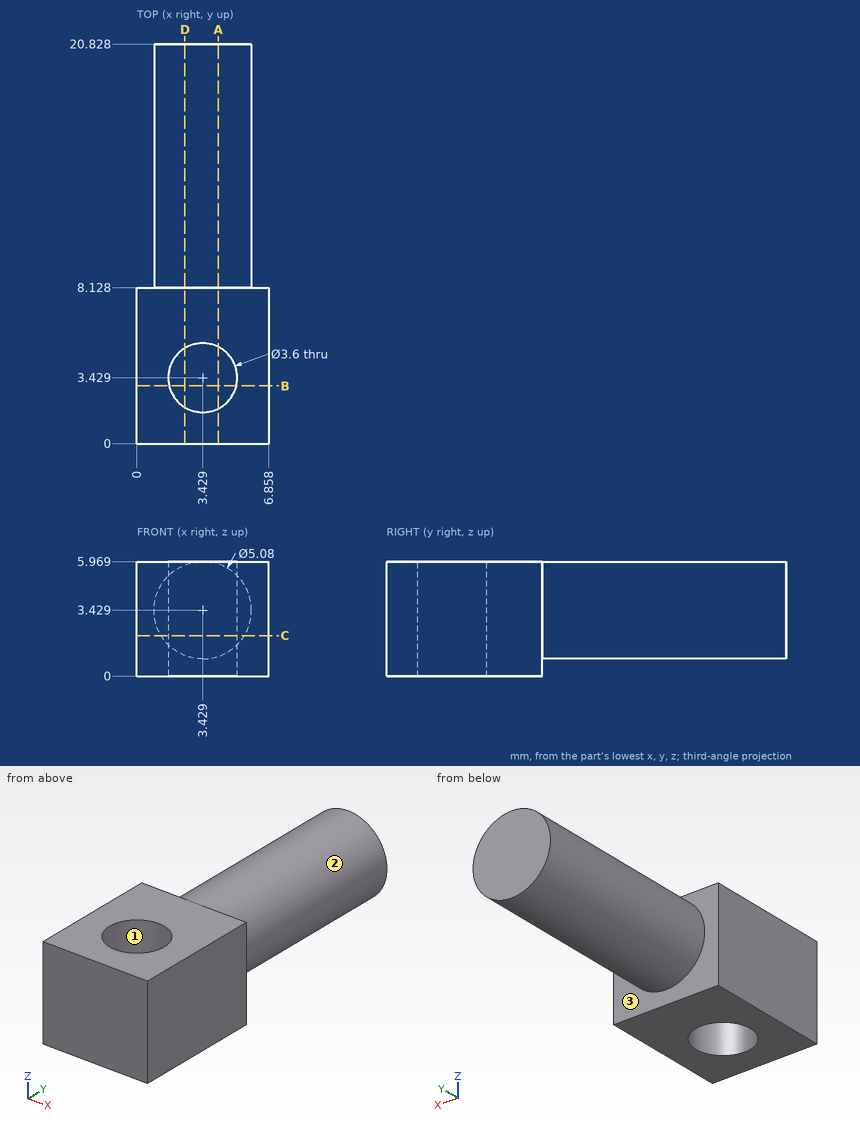
For this review, use the dimensioned drawing (mm, ordinates from the lowest corner) and the shaded views. Round coordinates to 2 decimals unless told otherwise and drop trailing zeros. Order: outer loops, then holes, each group sorted by start corner. A loop starts at its lowest first (then second) coordinate and runs counter-clockwise, first axis right, second up. Notation, with made-up numbers: (-10, 33.25) -> (38, 33.25) arc R22 ccw to (38, 70.25) -> close; hole circle Ø6 at (74.5, 53.5). An arc over 180 degrees is marked (long way). One line per item, written item: value. Start each with the question number.
Q1. Take a section at B-B (y = 3). Write out the cut boundary in (x, z).
Q2. Clearance check with flat-ended pins moving along their axes: pin 1 Ø4 at (x, y) = (4.5, 10) entering from +Z; pin 2 Ø2 at (x, y) = (5, 16.5) entering from -Z; pin 3 Ø1.5 at (y, z) = (17.5, 4.5) entering from +X; pin 4 Ø2 at (x, y) = (1.5, 10) entering from -Z (3 decimals). State where each tip first meets the part, or that it passes through.
Q3. Take a section at D-D (x = 2.5). Write out the cut boundary in (y, z).
Q4. Mouldability with a two-part tool opening along X and no side actions: class the marked faces 1, 2 and 3 as released by +X, released by -X, zero draft, split by the parting line, or undercut.
Q5. Take a section at A-A (x = 4.25). Write out the cut boundary in (y, z), and give its area (3 significant figures).
Q6. Take a section at C-C (z = 2.1). Write out the cut boundary in (x, y), and give its area (3 significant figures).
Q7. Wall thickness on line 1 (X direction, y = 3.5, z = 5.65); line 2 (Y direction, x = 0.5, z = 1.55); line 3 (Y direction, x = 4, z = 3.05): over which ranges is each line inside the solid? List them lowest first.
Reported:
1. outline: (0, 0) -> (1.68, 0) -> (1.68, 5.97) -> (0, 5.97) -> close; (5.18, 0) -> (6.86, 0) -> (6.86, 5.97) -> (5.18, 5.97) -> close
2. pin 1: stops at z = 5.97
2. pin 2: stops at z = 0.95
2. pin 3: stops at x = 5.95
2. pin 4: stops at z = 1.065
3. outline: (0, 0) -> (1.89, 0) -> (1.89, 5.97) -> (0, 5.97) -> close; (4.97, 0) -> (8.13, 0) -> (8.13, 1.06) -> (20.83, 1.06) -> (20.83, 5.79) -> (8.13, 5.79) -> (8.13, 5.97) -> (4.97, 5.97) -> close
4. face 1: undercut
4. face 2: split by the parting line
4. face 3: zero draft
5. outline: (0, 0) -> (1.83, 0) -> (1.83, 5.97) -> (0, 5.97) -> close; (5.03, 0) -> (8.13, 0) -> (8.13, 1.03) -> (20.83, 1.03) -> (20.83, 5.83) -> (8.13, 5.83) -> (8.13, 5.97) -> (5.03, 5.97) -> close
5. area: 90.4 mm2
6. outline: (0, 0) -> (6.86, 0) -> (6.86, 8.13) -> (5.59, 8.13) -> (5.59, 20.83) -> (1.26, 20.83) -> (1.26, 8.13) -> (0, 8.13) -> close; hole circle Ø3.6 at (3.43, 3.43)
6. area: 101 mm2
7. line 1: x = 0 to 1.63, 5.23 to 6.86
7. line 2: y = 0 to 8.13
7. line 3: y = 0 to 1.72, 5.14 to 20.83
